Verification items for the finished model (mm, model axes). A direction names the side the tool comes from. Coordinates: 2 decimals unless noted, no trailing zeros. Order: outer loops, then holes, each group sorted by start corner. A loop starts at its lowest first (then second) coordinate and runs counter-clockwise, first axis right, second up. Notation, with made-up numbers: M 20,-37 L 43,-37 A31 ccw 43,-1 Z; hole C 50.5,11 d10. An arc over 180 degrees is marked long. Return JSON: item names as keys, results as strings. Group by question number.
1. Section check D-D, the plane x = -74.5. Record the cut outline in (y, z).
2. Set-up check for faces 1 (the flat face through (82.136, 1, 27)), 2 (the flat face through (52.136, -17, 115)), 3 (the flat face through (67, 0, -80)), 4 (the flat face through (-113, 0, 130)), 5 (the flat face through (-24, 15, 24)): record each of +Z, -Z, +X, -X, +Y, -Y from which the full face is reachable in a straight line by a thin tool's end or side.
3. Section check A-A, the plane y = -17.5. Give the number of separate pieces and of enclosed holes in the cut face, plus the area to 3 significant figures.
4. Section check C-C, the plane z = 111. Record the cut outline in (x, y), plus the area to 3 significant figures.
5. Material ranges on line 1 along X through (y, z) = (-17, 113); line 2 along Z through (x, y) = (-100.5, -10.5); line 3 along Y through (x, z) = (-72, 63.5), recorded low to high.
6. Section check B-B, the plane x = 64. Record the cut outline in (y, z).
7. Gauge pin test, flat ends, axial feed: pin 1 (3 mm diameter, centred on x = 61, z = 132, fed in from +Y); pin 2 (16.5 mm diameter, centred on x = -18.5, y = 4.5, fed in from +Z); pin 3 (7.5 mm diameter, centred on x = -39, y = 4, fed in from -Z); pin 4 (1.5 mm diameter, centred on x = -102, y = -22.5, fed in from -Z). Record the tip position at first contact, or that the pin passes through.
8. Mould release check, pull along Z, two halves, no side actions. Record for faces 6 (the flat face through (67, 0, 130)), 7 (the flat face through (-126.41, -21.63, 135)), 8 (the flat face through (-126.41, -21.63, -45)): +Z half, -Z half, draft (parallel to the pull), parting line (faces both ways), or undercut.
```python
from build123d import *

# Parameters (mm, degrees)
IZIM1_W                     = 210
IZIM1_H                     = 200
Y_KSEKLIK_EKSTR_ZYON1_DEPTH = 15
IZIM2_W                     = 40
IZIM2_H                     = 35
Y_KSEKLIK_EKSTR_ZYON2_DEPTH = 30
IZIM7_R                     = 12.75
IZIM7_R_2                   = 14
KES_EKSTR_ZYON2_DEPTH       = 504


with BuildPart() as part:
    # Çizim1 → Yükseklik-Ekstrüzyon1 (new body)
    with BuildSketch(Plane(origin=(0, 0, 0), x_dir=(1, 0, 0), z_dir=(0, 1, 0))):
        with Locations((-22.864290172, -25)):
            Rectangle(IZIM1_W, IZIM1_H)
    extrude(amount=Y_KSEKLIK_EKSTR_ZYON1_DEPTH)

    # Çizim2 → Yükseklik-Ekstrüzyon2 (add)
    with BuildSketch(Plane(origin=(82.135709828, 0, 0), x_dir=(0, 0, -1), z_dir=(1, 0, 0))):
        with Locations((-115, -17.5)):
            Rectangle(IZIM2_W, IZIM2_H)
        with Locations((65, -17.5)):
            Rectangle(IZIM2_W, IZIM2_H)
    y_kseklik_ekstr_zyon2 = extrude(amount=-Y_KSEKLIK_EKSTR_ZYON2_DEPTH)

    # Aynalama1: Yükseklik-Ekstrüzyon2 across plane
    add(y_kseklik_ekstr_zyon2.mirror(Plane(origin=(-22.864290172, 0, 0), x_dir=(0, 0, 1), z_dir=(1, 0, 0))))

    # Çizim7 → Kes-Ekstrüzyon2 (cut)
    with BuildSketch(Plane.XY.offset(135)):
        with Locations((67.135709828, -17.5)):
            Circle(IZIM7_R)
        with Locations((-112.864290172, -17.5)):
            Circle(IZIM7_R_2)
    extrude(amount=-KES_EKSTR_ZYON2_DEPTH, mode=Mode.SUBTRACT)


solid = part.part
```
Answers follow:
{
 "1": {"outline": "M 0,-75 L 15,-75 L 15,125 L 0,125 Z"},
 "2": {"face 1": "+Z, -Z, +X, +Y, -Y", "face 2": "+Z, -Z, -Y", "face 3": "-Z, +X, -X, +Y", "face 4": "+Z, +X, -X, +Y", "face 5": "+Z, -Z, +X, -X, +Y"},
 "3": {"separate pieces": "8", "enclosed holes": "0", "area": "520 mm^2"},
 "4": {"outline": "M -127.86,-35 L -97.86,-35 L -97.86,0 L 52.14,0 L 52.14,-35 L 82.14,-35 L 82.14,15 L -127.86,15 Z; hole C -112.86,-17.5 d28; hole C 67.14,-17.5 d25.5", "area": "4,120 mm^2"},
 "5": {"line 1": "-127.86 to -126.86, -98.87 to -97.86, 52.14 to 54.4, 79.88 to 82.14", "line 2": "-85 to -45, 95 to 135", "line 3": "0 to 15"},
 "6": {"outline": "M -35,-85 L -29.86,-85 L -29.86,-45 L -35,-45 Z; M -35,95 L -29.86,95 L -29.86,135 L -35,135 Z; M -5.14,-85 L 0,-85 L 0,-75 L 15,-75 L 15,125 L 0,125 L 0,135 L -5.14,135 L -5.14,95 L 0,95 L 0,-45 L -5.14,-45 Z"},
 "7": {"pin 1": "y = 0", "pin 2": "z = 125", "pin 3": "z = -75", "pin 4": "through"},
 "8": {"face 6": "draft", "face 7": "+Z half", "face 8": "undercut"}
}
